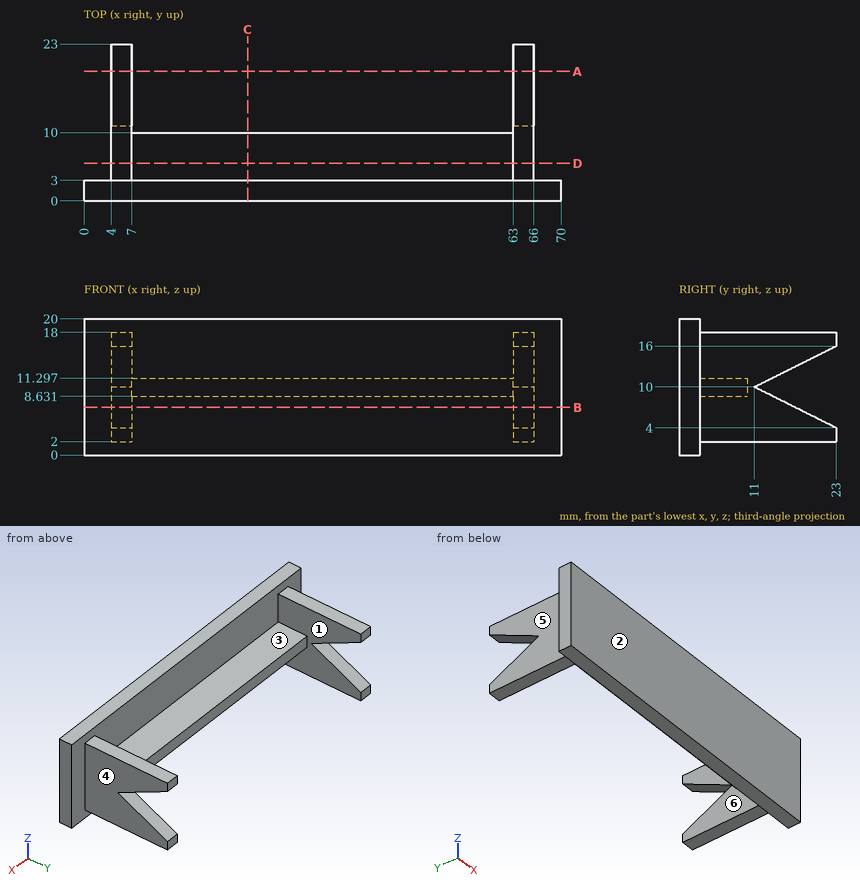
Part print with two shaded views. Sizes in mm from the minimum x, y, z corner. A direction names the side the tool comes from. Round coordinates to 2 decimals unless told otherwise and drop trailing zeros. Order: outer loops, then holes, each group sorted by start corner. A loop starts at its lowest first (then second) coordinate and runs counter-clockwise, first axis right, second up. Notation, with made-up numbers: (-7.5, 81) - (17.5, 81) arc R17 ccw to (17.5, 102) - close; hole circle Ø9 at (49, 11.25). An arc over 180 degrees is marked (long way). Answer in a Markdown table with one row per item. Add a question column.
(1) 3-axis set-ups, long thin cutter, end or side, ignore diameter. For the marked faces 1, 2 and 3: which of +Z, -Z, +X, -X, +Y, -Y reach the whole face in a straight line?
(2) Band-saw the part on C-C on x = 24. List the corners of the cut face in (y, z).
(3) Drop flat-ended pins along their axis: pin 1 Ø2.5 at (x, y) = (5.5, 16) entering from +Z; pin 2 Ø12 at (y, z) = (16.5, 10.5) entering from +X; pin 3 Ø1.5 at (x, y) = (64, 17) entering from -Z. Give the stop position or say it passes through.
(4) Band-saw the part on D-D on y = 5.5. List the corners of the cut face in (x, z).
(5) Probe L1, parallel to X at y = 17, z = 16.5; L2, parallel to Z at x = 46, y = 8.25; L3, parallel to Y at x = 7.5, z = 16.25. List the from-to ranges inside material, lowest first. Write a range as [from, to].
(6) Band-saw the part on A-A on y = 19. List the corners of the cut face in (x, z).
(7) Band-saw the part on B-B on z = 7. List the corners of the cut face in (x, y), and give its area (3 significant figures).
(8) Mould opens along X. For the marked faces 4, 5 and 6 say: +X half, -X half, draft (parallel to the pull), parting line (faces both ways), or undercut.
Data:
| question | item | result |
|---|---|---|
| 1 | face 1 | +Y |
| 1 | face 2 | +Z, -Z, +X, -X, -Y |
| 1 | face 3 | +Z, +Y |
| 2 | outline | (0, 0) - (3, 0) - (3, 8.63) - (10, 8.63) - (10, 11.3) - (3, 11.3) - (3, 20) - (0, 20) - close |
| 3 | pin 1 | stops at z = 18 |
| 3 | pin 2 | stops at x = 66 |
| 3 | pin 3 | stops at z = 2 |
| 4 | outline | (4, 2) - (7, 2) - (7, 8.63) - (63, 8.63) - (63, 2) - (66, 2) - (66, 18) - (63, 18) - (63, 11.3) - (7, 11.3) - (7, 18) - (4, 18) - close |
| 5 | L1 | x = [4, 7], [63, 66] |
| 5 | L2 | z = [8.63, 11.3] |
| 5 | L3 | y = [0, 3] |
| 6 | outline | (4, 2) - (7, 2) - (7, 6) - (4, 6) - close; (4, 14) - (7, 14) - (7, 18) - (4, 18) - close; (63, 2) - (66, 2) - (66, 6) - (63, 6) - close; (63, 14) - (66, 14) - (66, 18) - (63, 18) - close |
| 7 | outline | (0, 0) - (70, 0) - (70, 3) - (66, 3) - (66, 17) - (63, 17) - (63, 3) - (7, 3) - (7, 17) - (4, 17) - (4, 3) - (0, 3) - close |
| 7 | area | 294 mm^2 |
| 8 | face 4 | +X half |
| 8 | face 5 | -X half |
| 8 | face 6 | undercut |
